Could you check a few things on this model? Use its own coordinates, in mm. Face numbers are marked on the shaded views. Coordinates: 2 decimals unless noted, no trailing zeros. Loops run counter-clockwise (first coordinate to the right, second up) from the corner with the lowest first, then second, coordinate; pieces in that order, holes last. Notation, with made-up numbers: (52.25, 21) -> (66.25, 21) arc R25 ccw to (66.25, 49) -> close; hole circle Ø5 at (14, 32.25). An arc over 180 degrees is marked (long way). One line per question, with ' | ' between items. Start each with the question number.
(1) Suppose I cut it at B-B (x = 9). Please give me the cut outline in (y, z).
(2) Suppose I cut it at A-A (z = 2). Please give me the cut outline in (x, y), plus the area to 3 significant figures.
(3) If I drill on line 1 along X through (y, z) = (-5.5, -0.5); line 2 along X through (y, z) = (-5, 1); line 3 along X through (y, z) = (-10.75, -2.5), over which ranges is the centre line in solid material (lowest first)?
(4) Suppose I cut it at D-D (x = -13). Please give me the cut outline in (y, z), plus the area to 3 significant figures.
(5) I'm going to push flat-ended pins straight in: pin 1 Ø4 at (x, z) = (8.42, 0) entering from +Y; pin 2 Ø2 at (x, y) = (-14, -7) entering from -Z. Where does each tip first touch, or does it pass through?
(6) If we mould it in two halves opening along Z, with no side actions, what happens to the marked faces 1, 2 and 3? For each: pulls with the +Z half, pulls with the -Z half, needs draft (parallel to the pull), parting line crosses it, or undercut.
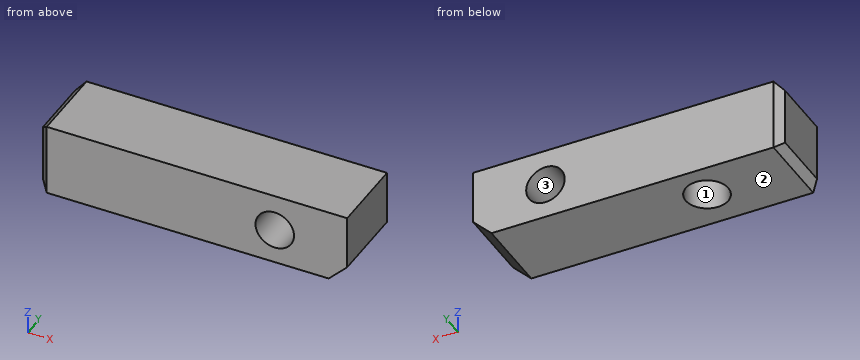
```python
from build123d import *

# Parameters (mm, degrees)
F0_W     = 50.8
F0_H     = 11.938
F1_DEPTH = 12.7
F2_R     = 3.175
F3_DEPTH = 12.701
F5_DEPTH = 6.35
F6_SIZE  = 3.048
F7_SIZE  = 1.27


with BuildPart() as f1:
    # F0 (on Front) → F1 (new body)
    with BuildSketch(Plane.XZ):
        with Locations((-5.045198, 0.153461)):
            Rectangle(F0_W, F0_H)
    extrude(amount=F1_DEPTH)

    # F2 (on face) → F3 (cut, through all)
    with BuildSketch(Plane.XZ.offset(12.7)):
        with Locations((8.416499, 0)):
            Circle(F2_R)
    extrude(amount=-F3_DEPTH, mode=Mode.SUBTRACT)

    # F4 (on Top) → F5 (cut)
    with BuildSketch(Plane.XY):
        with BuildLine():
            ThreePointArc((-18.664943, -5.920342), (-15.166093, -9.419192), (-11.667243, -5.920342))
            ThreePointArc((-11.667243, -5.920342), (-15.166093, -2.421492), (-18.664943, -5.920342))
        make_face()
    extrude(amount=-F5_DEPTH, mode=Mode.SUBTRACT)

    # F6
    f6_edges = [f1.edges().sort_by_distance(p)[0] for p in [
        (20.354802, -6.35, -5.815539),
    ]]
    chamfer(f6_edges, length=F6_SIZE)

    # F7
    f7_edges = [f1.edges().sort_by_distance(p)[0] for p in [
        (-30.445198, -6.35, 6.122461),
        (-30.445198, -12.7, 0.153461),
        (-30.445198, -6.35, -5.815539),
        (-30.445198, 0, 0.153461),
    ]]
    chamfer(f7_edges, length=F7_SIZE)


solid = f1.part
```
Checks:
1) outline: (-12.7, -5.82) -> (0, -5.82) -> (0, -3.12) -> (-12.7, -3.12) -> close; (-12.7, 3.12) -> (0, 3.12) -> (0, 6.12) -> (-12.7, 6.12) -> close
2) outline: (-30.45, -11.43) -> (-29.18, -12.7) -> (5.95, -12.7) -> (5.95, 0) -> (-29.18, 0) -> (-30.45, -1.27) -> close; (10.88, -12.7) -> (20.35, -12.7) -> (20.35, 0) -> (10.88, 0) -> close | area: 581 mm^2
3) line 1: x = -30.45 to -18.64, -11.69 to 5.28, 11.55 to 20.35 | line 2: x = -30.45 to 5.4, 11.43 to 20.35 | line 3: x = -30.45 to 6.46, 10.37 to 20.35
4) outline: (-12.7, -5.82) -> (-8.67, -5.82) -> (-8.67, 0) -> (-3.17, 0) -> (-3.17, -5.82) -> (0, -5.82) -> (0, 6.12) -> (-12.7, 6.12) -> close | area: 120 mm^2
5) pin 1: passes through | pin 2: stops at z = 0
6) face 1: needs draft | face 2: pulls with the -Z half | face 3: undercut
